Model file for the job. Use its own axes, mm. Face numbers are marked on the shaded views. A direction names the side the tool comes from. Round coordinates to 2 decimals unless told otherwise and drop trailing zeros. Write each loop counter-clockwise with the first axis right and the second up, starting at its lowest first coordinate (ties: lowest second). Pieces come first, ordered by that corner, then holes.
```python
from build123d import *

# Parameters (mm, degrees)
SKETCH_1_R          = 1.5
SKETCH_1_R_2        = 1
EXTRUDE_2_DEPTH     = 2.4
SKETCH_2_W          = 1.9
SKETCH_2_H          = 20
SKETCH_2_W_2        = 2
EXTRUDE_3_DEPTH     = 10
CUT_EXTRUDE_1_DEPTH = 15
CUT_EXTRUDE_2_DEPTH = 20
SKETCH_8_W          = 13.9
SKETCH_8_H          = 20.615528128
EXTRUDE_5_DEPTH     = 2
SKETCH_9_R          = 3.5
CUT_EXTRUDE_4_DEPTH = 2
CUT_EXTRUDE_5_DEPTH = 20


with BuildPart() as part:
    # 草图1 → 凸台-拉伸2 (new body)
    with BuildSketch(Plane.XY):
        with BuildLine():
            Line((14.436511473, 15.948106541), (20.186511473, 15.948106541))
            Line((20.186511473, 15.948106541), (20.186511473, 25.081955572))
            ThreePointArc((20.186511473, 25.081955572), (25.186511473, 30.081955572), (30.186511473, 25.081955572))
            Line((30.186511473, 25.081955572), (30.186511473, 15.948106541))
            Line((30.186511473, 15.948106541), (35.936511473, 15.948106541))
            add(Edge.make_bspline(
                [(39.436511473, 18.679045823), (39.436511473, 17.199254946), (37.41630235, 15.948106541), (35.936511473, 15.948106541)],
                knots=[0, 0, 0, 0, 4.439372631, 4.439372631, 4.439372631, 4.439372631], degree=3))
            Line((39.436511473, 18.679045823), (39.436511473, 22.179045823))
            Line((39.436511473, 22.179045823), (33.686511473, 40.132696196))
            Line((33.686511473, 40.132696196), (25.186511473, 40.132696196))
            Line((25.186511473, 40.132696196), (16.686511473, 40.132696196))
            Line((16.686511473, 40.132696196), (10.936511473, 22.179045823))
            Line((10.936511473, 22.179045823), (10.936511473, 18.679045823))
            add(Edge.make_bspline(
                [(10.936511473, 18.679045823), (10.936511473, 17.199254946), (12.956720596, 15.948106541), (14.436511473, 15.948106541)],
                knots=[0, 0, 0, 0, 4.439372631, 4.439372631, 4.439372631, 4.439372631], degree=3))
        make_face()
        with Locations((14.436511473, 22.132696196)):
            Circle(SKETCH_1_R, mode=Mode.SUBTRACT)
        with Locations((35.936511473, 22.132696196)):
            Circle(SKETCH_1_R, mode=Mode.SUBTRACT)
        with Locations((27.936511473, 35.132696196)):
            Circle(SKETCH_1_R_2, mode=Mode.SUBTRACT)
        with Locations((22.436511473, 35.132696196)):
            Circle(SKETCH_1_R_2, mode=Mode.SUBTRACT)
    extrude(amount=EXTRUDE_2_DEPTH)

    # 草图2 → 凸台-拉伸3 (add)
    with BuildSketch(Plane.XY.offset(2.4)):
        with Locations((31.136511473, 20.948106541)):
            Rectangle(SKETCH_2_W, SKETCH_2_H)
        with Locations((19.186511473, 20.948106541)):
            Rectangle(SKETCH_2_W_2, SKETCH_2_H)
    extrude(amount=EXTRUDE_3_DEPTH)

    # 草图4 → 切除-拉伸1 (cut)
    with BuildSketch(Plane.ZY.offset(-18.186511473)):
        Polygon((2.4, 15.948106541), (7.4, 10.948106541), (2.4, 10.948106541), align=None)
    extrude(amount=-CUT_EXTRUDE_1_DEPTH, mode=Mode.SUBTRACT)

    # 草图5 → 切除-拉伸2 (cut)
    with BuildSketch(Plane.ZY.offset(-18.186511473)):
        Polygon((12.4, 10.948106541), (12.4, 30.948106541), (7.4, 10.948106541), align=None)
    extrude(amount=-CUT_EXTRUDE_2_DEPTH, mode=Mode.SUBTRACT)

    # 草图8 → 凸台-拉伸5 (add)
    with BuildSketch(Plane(origin=(0, -1.097170203, 4.388680814), x_dir=(1, 0, 0), z_dir=(0, -0.242535625, 0.9701425))):
        with Locations((25.136511473, 22.723751141)):
            Rectangle(SKETCH_8_W, SKETCH_8_H)
    extrude(amount=EXTRUDE_5_DEPTH)

    # 草图9 → 切除-拉伸4 (cut)
    with BuildSketch(Plane(origin=(0, -1.582241454, 6.328965814), x_dir=(1, 0, 0), z_dir=(0, -0.242535625, 0.9701425))):
        with Locations((25.136511473, 19.304044077)):
            Circle(SKETCH_9_R)
    extrude(amount=-CUT_EXTRUDE_4_DEPTH, mode=Mode.SUBTRACT)

    # 草图10 → 切除-拉伸5 (cut)
    with BuildSketch(Plane.ZY.offset(-18.186511473)):
        Polygon((2.4, 30.948106541), (12.541594878, 23.268274803), (18.273865584, 30.948106541), align=None)
    extrude(amount=-CUT_EXTRUDE_5_DEPTH, mode=Mode.SUBTRACT)


solid = part.part
```
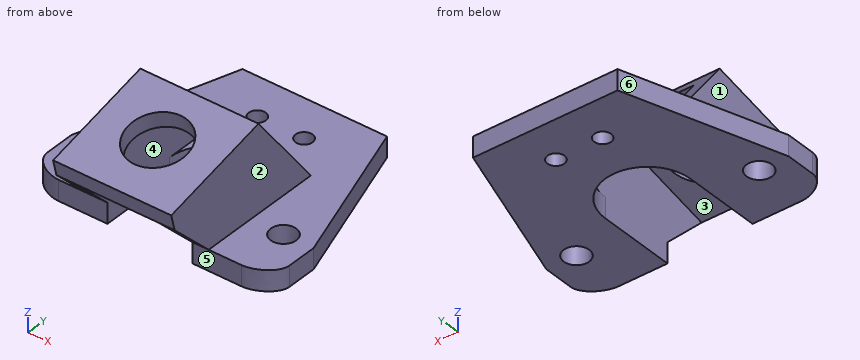
1) Flat gauge pins, fed straight in: pin 1 Ø3 at (x, y) = (17.5, 19.5) entering from +Z; pin 2 Ø2.5 at (x, y) = (35.94, 22.13) entering from -Z; pin 3 Ø1 at (x, y) = (19, 29.5) entering from +Z; pin 4 Ø0.7 at (x, z) = (18, 1.5) entering from -Y. Where does each tip first touch, or does it go through?
2) Cut at B-B on x = 25.5. List the corners of the cut face in (y, z).
3) Which spindle directions (+Z, -Z, +X, -X, +Y, -Y) get a long thin tool onto all of the face, cutting with end or side? Do the marked faces 1, 2 and 3. Say none if no direction does.
4) Cut at D-D on x = 19.25. List the corners of the cut face in (y, z), and give its area (3 significant figures).
5) Wall check: probe 1 along X at (y, z) = (14, 5.5); probe 2 along Z at (x, y) = (20.25, 27.75); probe 3 along X at (y, z) = (13.25, 8.25). Give the ranges that are in metal, low to high.
6) Cut at A-A on z = 3.5. List the corners of the cut face in (x, y).
7) Cut at C-C on y = 28. List the corners of the cut face in (x, z).
8) Pull direction X, two halves, no side cores. Call the marked faces 4, 5 and 6: released by +X, released by -X, zero draft, split by the parting line, or undercut.
Result sheet:
1. pin 1: stops at z = 11.93
1. pin 2: passes through
1. pin 3: stops at z = 4.97
1. pin 4: stops at y = 15.95
2. outline: (10.46, 9.34) - (10.95, 7.4) - (14.25, 8.23) - (13.77, 10.17) - close; (20.52, 11.86) - (21.01, 9.91) - (24.58, 10.81) - (23.27, 12.54) - close; (30.07, 0) - (40.13, 0) - (40.13, 2.4) - (30.07, 2.4) - close
3. face 1: +Z, -X, +Y, -Y
3. face 2: +Z, +X, +Y, -Y
3. face 3: -Z, +Y
4. outline: (10.46, 9.34) - (10.95, 7.4) - (15.95, 2.4) - (15.95, 0) - (40.13, 0) - (40.13, 2.4) - (30.95, 2.4) - (23.27, 12.54) - close
4. area: 191 mm2
5. probe 1: x = 18.19 to 20.19, 30.19 to 32.09
5. probe 2: z = 0 to 2.4
5. probe 3: x = 18.19 to 32.09
6. outline: (18.19, 14.85) - (20.19, 14.85) - (20.19, 30.12) - (18.19, 30.12) - close; (30.19, 14.85) - (32.09, 14.85) - (32.09, 30.12) - (30.19, 30.12) - close
7. outline: (12.8, 0) - (21.13, 0) - (21.13, 2.4) - (20.19, 2.4) - (20.19, 6.29) - (18.19, 6.29) - (18.19, 2.4) - (12.8, 2.4) - close; (29.25, 0) - (37.57, 0) - (37.57, 2.4) - (32.09, 2.4) - (32.09, 6.29) - (30.19, 6.29) - (30.19, 2.4) - (29.25, 2.4) - close
8. face 4: undercut
8. face 5: zero draft
8. face 6: released by -X
